The listing builds one solid part. Answer for the finished solid, in the listing's coordinates (mm). Face numbers are marked on the shaded views. A direction names the side the tool comes from. Round coordinates to 2 decimals unless told otherwise and drop trailing zeros. Write each loop counter-clockwise with the first axis right and the second up, starting at its lowest first coordinate (ties: lowest second). Pieces come first, ordered by that corner, then holes.
(1) Each of these flat-tipped pins is pushed along its axis until it touches: pin 1 Ø1 at (x, y) = (-7.5, -6.5) entering from +Z; pin 2 Ø2 at (x, y) = (-1, -21) entering from +Z; pin 3 Ø7 at (x, y) = (2.5, -18.5) entering from -Z (3 decimals). Where does it stop, or does it pass through?
(2) The mould has two halves that part along Y. Classify the marked faces 1, 2 and 3: +Y half, -Y half, draft (parallel to the pull), parting line (faces both ways), or undercut.
(3) Find the intervals of material crossed by probe 1 along Y at (x, z) = (-7.5, -2.25) (3 decimals); probe 2 along X at (y, z) = (13, -9); probe 3 along Z at (x, y) = (-10.5, 10.5), in increasing order.
(4) A cutting plane is placed at A-A, the plane z = -1.5. Give the vertices of the cut face in (x, y) (1 decimal), and give its area (3 significant figures).
(5) A cutting plane is placed at C-C, the plane z = -9.5. Give the number of separate pieces and of enclosed holes in the cut face, and give its area (3 significant figures).
(6) For the marked faces 4, 5 and 6, determine the directions among +Z, -Z, +X, -X, +Y, -Y from which every point of the face is accessible in a straight line to the end or side of a thin tool.
(7) A cutting plane is placed at B-B, the plane y = 2.5. Give the vertices of the cut face in (x, z).
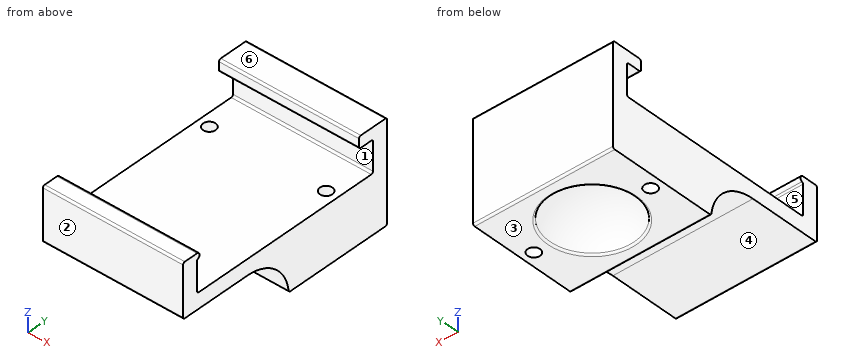
from build123d import *

# Parameters (mm, degrees)
BOSS_EXTRUDE1_DEPTH = 14.2875
FILLET1_R           = 0.396875
BOSS_EXTRUDE2_DEPTH = 14.2875
FILLET2_R           = 0.396875
SKETCH5_R           = 1.27
CUT_EXTRUDE1_DEPTH  = 12.7
FILLET3_R           = 9.525


with BuildPart() as part:
    # Sketch2 → Boss-Extrude1 (new body, symmetric)
    with BuildSketch(Plane(origin=(0, 0, 0), x_dir=(0, 0, -1), z_dir=(1, 0, 0))):
        with BuildLine():
            Line((-3.25, 16.825), (-5.63125, 16.825))
            Line((-5.63125, 16.825), (-5.63125, 23.175))
            Line((-5.63125, 23.175), (6.425, 23.175))
            Line((6.425, 23.175), (6.425, -23.175))
            Line((6.425, -23.175), (-4.440625, -23.175))
            Line((-4.440625, -23.175), (-4.440625, -20))
            ThreePointArc((-4.440625, -20), (-3.8453125, -19.4046875), (-3.25, -20))
            Line((-3.25, -20), (3.25, -20))
            Line((3.25, -20), (3.25, 20))
            Line((3.25, 20), (-3.25, 20))
            Line((-3.25, 20), (-3.25, 16.825))
        make_face()
    extrude(amount=BOSS_EXTRUDE1_DEPTH, both=True)

    # Fillet1
    fillet1_edges = [part.edges().sort_by_distance(p)[0] for p in [
        (0, 20, -3.25),
        (0, 20, 3.25),
        (0, 16.825, 3.25),
        (0, 16.825, 5.63125),
        (0, 23.175, 5.63125),
        (0, -23.175, 4.440625),
        (0, -20, 3.25),
        (0, -20, -3.25),
    ]]
    fillet(fillet1_edges, radius=FILLET1_R)

    # Sketch3 → Boss-Extrude2 (add, symmetric)
    with BuildSketch(Plane(origin=(0, 0, 0), x_dir=(0, 0, -1), z_dir=(1, 0, 0))):
        Polygon((6.425, 23.175), (15.061, 23.175), (15.061, 20.635), (15.061, 3.363), (15.061, 0.823), (6.425, 0.823), align=None)
    extrude(amount=BOSS_EXTRUDE2_DEPTH, both=True)

    # Sketch4 → Cut-Revolve3 (revolve, cut)
    with BuildSketch(Plane(origin=(0, 0, 0), x_dir=(0, 0, -1), z_dir=(1, 0, 0))):
        with BuildLine():
            Line((15.061, 3.363), (15.061, 20.635))
            ThreePointArc((15.061, 20.635), (6.425, 11.999), (15.061, 3.363))
        make_face()
    revolve(axis=Axis((0, 3.363, -15.061), (0, 1, 0)), mode=Mode.SUBTRACT)

    # Fillet2
    fillet2_edges = [part.edges().sort_by_distance(p)[0] for p in [
        (0, -23.175, -6.425),
        (0, 23.175, -15.061),
        (0, 0.823, -15.061),
        (8.636, 11.999, -15.061),
    ]]
    fillet(fillet2_edges, radius=FILLET2_R)

    # Sketch5 → Cut-Extrude1 (cut)
    with BuildSketch(Plane(origin=(0, 0, -15.061), x_dir=(-1, 0, 0), z_dir=(0, 0, -1))):
        with Locations((-11.90625, 11.999)):
            Circle(SKETCH5_R)
        with Locations((11.90625, 11.999)):
            Circle(SKETCH5_R)
    extrude(amount=-CUT_EXTRUDE1_DEPTH, mode=Mode.SUBTRACT)

    # Fillet3
    fillet3_edges = [part.edges().sort_by_distance(p)[0] for p in [
        (0, 0.823, -6.425),
    ]]
    fillet(fillet3_edges, radius=FILLET3_R)


solid = part.part
Solutions:
1. pin 1: stops at z = -3.25
1. pin 2: stops at z = 4.44
1. pin 3: stops at z = -6.425
2. face 1: undercut
2. face 2: -Y half
2. face 3: draft
3. probe 1: y = -23.175 to -20, 20 to 23.175
3. probe 2: x = -14.29 to -12.69, -11.12 to -6.07, 6.07 to 11.12, 12.69 to 14.29
3. probe 3: z = -15.06 to -3.25
4. outline: (-14.3, -23.2) - (14.3, -23.2) - (14.3, -20) - (-14.3, -20) - close; (-14.3, 20) - (14.3, 20) - (14.3, 23.2) - (-14.3, 23.2) - close
4. area: 181 mm2
5. separate pieces: 1
5. enclosed holes: 3
5. area: 561 mm2
6. face 4: -Z, +X, -X, -Y
6. face 5: +X, -X
6. face 6: +Z, +X, -X, +Y, -Y
7. outline: (-14.29, -15.06) - (14.29, -15.06) - (14.29, -3.25) - (-14.29, -3.25) - close
